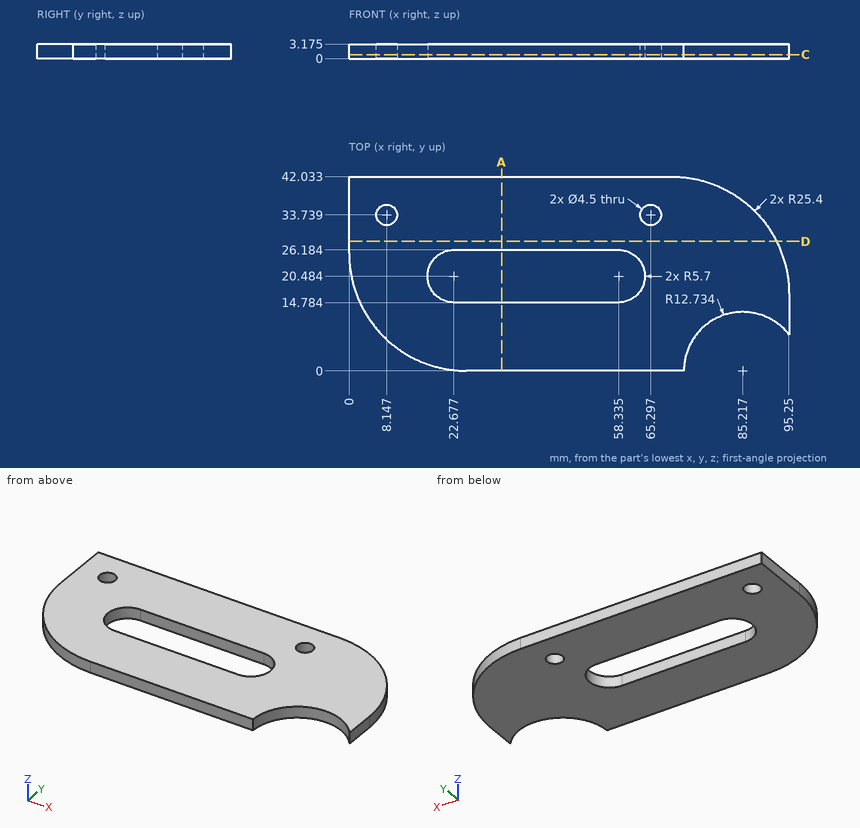
Print and shaded views of the part. All mm, measured from the part's lowest x, y and z. Give positions to 0.01 mm unless a question says otherwise; leave off trailing zeros. Loops run counter-clockwise (first coordinate to the right, second up) from the corner with the lowest first, then second, coordinate; pieces in that order, holes last. Notation, with made-up numbers: M 13,27.5 L 55,27.5 A35 ccw 55,64.5 Z; hole C 35,66 d6. An arc over 180 degrees is marked long. Write each question's results on one line, items separated by ' | '.
Q1. Probe probe 1 along Y at (x, z) = (49, 2); probe 2 along X at (y, z) = (35, 0.25) (1 decimal); probe 3 along X at (y, z) = (21, 1.45) (1 decimal). List the from-to ranges inside material, lowest first.
Geometry check:
probe 1: y = 0 to 14.78, 26.18 to 42.03 | probe 2: x = 0 to 6.3, 10 to 63.4, 67.2 to 87.4 | probe 3: x = 0.4 to 17, 64 to 94.9
Q2. Flat gauge pin, fed straight in: P1, Ø1.5, axis at y = 31, z = 2.5, coming from the +X side. Where does the tip first touch, or does it go through?
Geometry check:
P1: stops at x = 91.29
Q3. Band-saw the part on D-D on y = 28. Write the cut outline in (x, z) (1 decimal).
Geometry check:
outline: M 0,0 L 92.6,0 L 92.6,3.2 L 0,3.2 Z
Q4. Band-saw the part on C-C on z = 0.9. Give the number of separate pieces and of enclosed holes in the cut face, and give its area (3 significant figures).
Geometry check:
separate pieces: 1 | enclosed holes: 3 | area: 2,950 mm²
Q5. Band-saw the part on A-A on x = 33. Write the cut outline in (y, z) (1 decimal).
Geometry check:
outline: M 0,0 L 14.8,0 L 14.8,3.2 L 0,3.2 Z; M 26.2,0 L 42,0 L 42,3.2 L 26.2,3.2 Z
